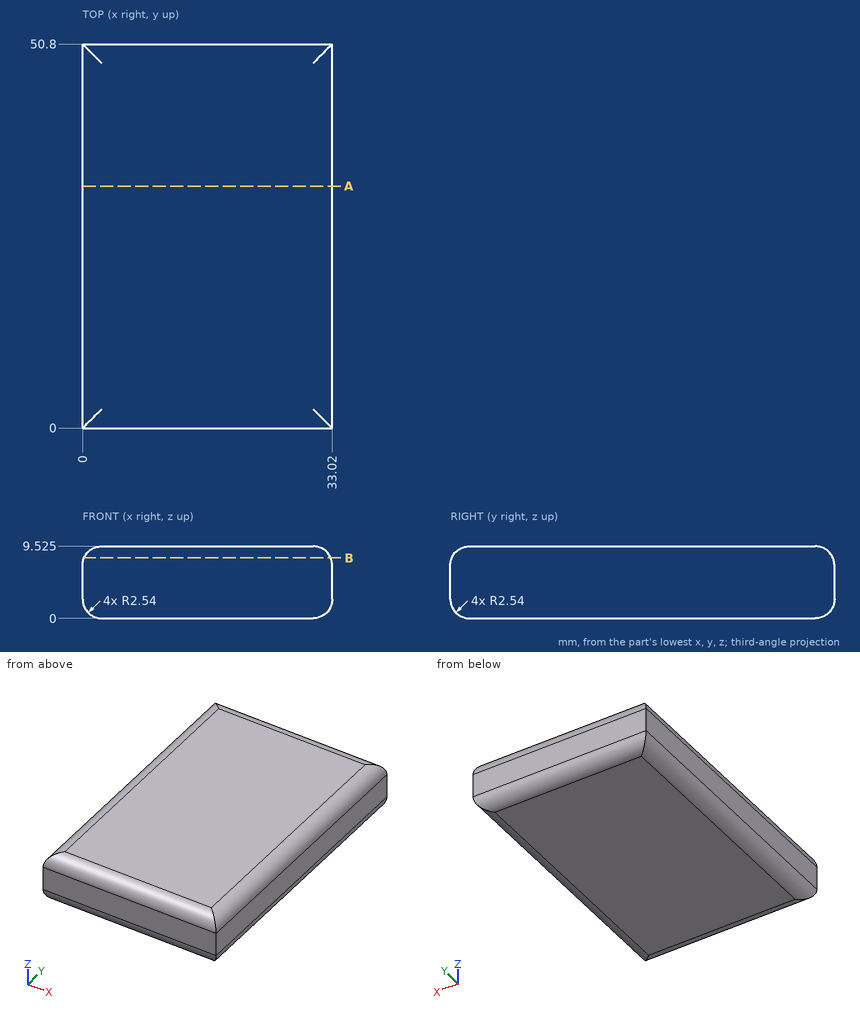
Could you check a few things on this drawing? It's one solid part, dimensions in mm from its lowest x, y, z. Give positions to 0.01 mm unless a question says otherwise; leave off trailing zeros. Write each loop counter-clockwise with the first axis right and the second up, starting at its lowest first coordinate (ties: lowest second). Pieces come first, ordered by that corner, then holes. Notation, with made-up numbers: (-37, 42) -> (-23, 42) arc R10 ccw to (-23, 59) -> close; hole circle Ø3 at (52, 52.25). An arc over 180 degrees is marked (long way). Write each question's results on one line, items separated by ' | '.
1. I need wall thicknesses on L1, parallel to Y at x = 18, z = 1.5; L2, parallel to Y at x = 4, z = 8.75; L3, parallel to X at y = 16, z = 8. Which ranges of each line are inside material? Lowest first, please.
Check sheet entries:
L1: y = 0.22 to 50.58 | L2: y = 0.71 to 50.09 | L3: x = 0.21 to 32.81
2. I want a section at A-A, the plane y = 32. Write out the boundary of the cut face in (x, z) (3 decimals).
Check sheet entries:
outline: (0, 2.54) arc R2.54 ccw to (2.54, 0) -> (30.48, 0) arc R2.54 ccw to (33.02, 2.54) -> (33.02, 6.985) arc R2.54 ccw to (30.48, 9.525) -> (2.54, 9.525) arc R2.54 ccw to (0, 6.985) -> close
3. I want a section at B-B, the plane z = 8. Write out the boundary of the cut face in (x, y).
Check sheet entries:
outline: (0.21, 0.21) -> (32.81, 0.21) -> (32.81, 50.59) -> (0.21, 50.59) -> close
4. Will this pin go through, and if not, where does the flat tip stop? pin 1 Ø1 at (x, y) = (8.5, 9) entering from -Z.
Check sheet entries:
pin 1: stops at z = 0
